Autodesk Inventor part; units mm, degrees
ref_plane "YZ Plane" through (0, 0, 0) normal (1, 0, 0) x (0, 1, 0)
ref_plane "XZ Plane" through (0, 0, 0) normal (0, 1, 0) x (-1, 0, 0)
ref_plane "XY Plane" through (0, 0, 0) normal (0, 0, 1) x (1, 0, 0)
sketch "Sketch1" plane through (0, 0, 0) normal (0, 0, 1) x (1, 0, 0)
  line L0 (0, 0) -> (45.5, 0)
  line L1 (45.5, 0) -> (45.5, 10)
  line L2 (45.5, 10) -> (0, 10)
  line L3 (0, 10) -> (0, 0)
  dimension "d0" = 45.5
  dimension "d1" = 10
extrude "Extrusion1" add sketch "Sketch1" along normal blind 3
sketch "Sketch2" plane through (0, 0, 3) normal (0, 0, 1) x (1, 0, 0)
  line L0 (0, 10) -> (0, 0)
  line L1 (45.5, 0) -> (45.5, 10)
  line L2 (45.5, 10) -> (0, 10)
  point P0 (7, 5)
  point P1 (38.5, 5)
  dimension "d4" = 7
  dimension "d5" = 7
  dimension "d6" = 5
  dimension "d7" = 5
sketch "Sketch3" plane through (0, 0, 3) normal (0, 0, 1) x (1, 0, 0)
  point P0 (0, 0)
hole "Hole1" at (7, 5, 3) at (38.5, 5, 3) direction (0, 0, -1) diameter 4.4 end through all
properties part number "pipeServo"
Could you check a few things on this model? Use its own coordinates, in mm. Round coordinates to 2 decimals unless told otherwise and drop trailing zeros. Write each loop counter-clockwise with the first axis right and the second up, starting at its lowest first coordinate (ties: lowest second). Pieces come first, ordered by that corner, then holes. Notation, with made-up numbers: M -25.75,79.25 L 14.25,79.25 A13 ccw 14.25,103.25 Z; hole C 27,63 d7. An arc over 180 degrees is marked long. Answer in a Markdown table with one row per item. Add a question column.
Q1. Imagine slicing it at C-C (z = 0.95). Please give me the cut outline in (x, y), then the cut area to 3 significant figures.
Q2. Imagine slicing it at A-A (y = 5). Please give me the cut outline in (x, z).
Q3. If I drill on line 1 (X direction, y = 5, z = 1.9); line 2 (Y direction, x = 7, z = 0.85); line 3 (X direction, y = 6, z = 1.45), over which ranges is the centre line in solid material (lowest first)? Write a range as from..to.
Q4. Imagine slicing it at B-B (x = 7). Please give me the cut outline in (y, z), then the cut area to 3 significant figures.
Q5. Will this pin go through, and if not, where does the flat tip stop? pin 1 Ø1.5 at (y, z) = (9, 2.5) entering from -X.
Q6. If we mould it in two halves opening along X, with no side actions, what happens to faces 1 (the cylindrical face through (40.648, 5.477, 1.479)), 2 (the cylindrical face through (6.34, 2.9, 1.48)), 3 (the flat face through (45.5, 5, 1)), 4 (the flat face through (22, 5, 3))? For each: +X half, -X half, draft (parallel to the pull), parting line (faces both ways), or undercut.
Values:
| question | item | result |
|---|---|---|
| 1 | outline | M 0,0 L 45.5,0 L 45.5,10 L 0,10 Z; hole C 7,5 d4.4; hole C 38.5,5 d4.4 |
| 1 | area | 425 mm^2 |
| 2 | outline | M 0,0 L 4.8,0 L 4.8,3 L 0,3 Z; M 9.2,0 L 36.3,0 L 36.3,3 L 9.2,3 Z; M 40.7,0 L 45.5,0 L 45.5,3 L 40.7,3 Z |
| 3 | line 1 | 0..4.8, 9.2..36.3, 40.7..45.5 |
| 3 | line 2 | 0..2.8, 7.2..10 |
| 3 | line 3 | 0..5.04, 8.96..36.54, 40.46..45.5 |
| 4 | outline | M 0,0 L 2.8,0 L 2.8,3 L 0,3 Z; M 7.2,0 L 10,0 L 10,3 L 7.2,3 Z |
| 4 | area | 16.8 mm^2 |
| 5 | pin 1 | x = 0 |
| 6 | face 1 | undercut |
| 6 | face 2 | undercut |
| 6 | face 3 | +X half |
| 6 | face 4 | draft |
